from build123d import *

# Parameters (mm, degrees)
SKETCH_2_W          = 10
SKETCH_2_H          = 8
EXTRUDE_1_DEPTH     = 12.5
SKETCH_3_W          = 10
SKETCH_3_H          = 5
CUT_EXTRUDE_1_DEPTH = 10
SKETCH_4_R          = 1.6
CUT_EXTRUDE_2_DEPTH = 18.895530168
SKETCH_5_OUTSIDE_W  = 15.58
SKETCH_5_OUTSIDE_H  = 18.08
CUT_EXTRUDE_3_DEPTH = 18.895530168


with BuildPart() as part:
    # ｽｹｯﾁ2 → ﾎﾞｽ - 押し出し1 (new body)
    with BuildSketch(Plane(origin=(0, 0, 0), x_dir=(1, 0, 0), z_dir=(0, 1, 0))):
        with Locations((5, 4)):
            Rectangle(SKETCH_2_W, SKETCH_2_H)
    extrude(amount=EXTRUDE_1_DEPTH)

    # ｽｹｯﾁ3 → ｶｯﾄ - 押し出し1 (cut)
    with BuildSketch(Plane(origin=(0, 12.5, 0), x_dir=(1, 0, 0), z_dir=(0, 1, 0))):
        with Locations((5, 4)):
            Rectangle(SKETCH_3_W, SKETCH_3_H)
    extrude(amount=-CUT_EXTRUDE_1_DEPTH, mode=Mode.SUBTRACT)

    # ｽｹｯﾁ4 → ｶｯﾄ - 押し出し2 (cut, through all)
    with BuildSketch(Plane.XY):
        with Locations((5, 7.5)):
            Circle(SKETCH_4_R)
    extrude(amount=-CUT_EXTRUDE_2_DEPTH, mode=Mode.SUBTRACT)

    # ｽｹｯﾁ5 outside → ｶｯﾄ - 押し出し3 (cut, through all)
    with BuildSketch(Plane.XY):
        with Locations((5, 6.25)):
            Rectangle(SKETCH_5_OUTSIDE_W, SKETCH_5_OUTSIDE_H)
        with BuildLine():
            Line((0, 7.5), (0, 0))
            Line((0, 0), (10, 0))
            Line((10, 0), (10, 7.5))
            ThreePointArc((10, 7.5), (5, 12.5), (0, 7.5))
        make_face(mode=Mode.SUBTRACT)
    extrude(amount=-CUT_EXTRUDE_3_DEPTH, mode=Mode.SUBTRACT)


solid = part.part
Geometry: final body of the model. Coordinates: model frame, mm. A direction names the side the tool comes from. Give positions to 0.01 mm unless a question says otherwise; leave off trailing zeros. Write each loop counter-clockwise with the first axis right and the second up, starting at its lowest first coordinate (ties: lowest second). Pieces come first, ordered by that corner, then holes. Notation, with made-up numbers: (-1.5, -24) -> (53.5, -24) arc R26 cw to (53.5, 0) -> close; hole circle Ø7 at (4, 0). An arc over 180 degrees is marked (long way). Answer in a Markdown table with one row per item.
(1) Ray query, line 1 along Z through (x, y) = (1.25, 10.25); line 2 along Y through (x, z) = (5, -0.35); line 3 along Y through (x, z) = (1.75, -4). Return the intervals inside material, ascending. Write a range as [from, to].
Answers below:
| item | result |
|---|---|
| line 1 | [-8, -6.5], [-1.5, 0] |
| line 2 | [0, 5.9], [9.1, 12.5] |
| line 3 | [0, 2.5] |
(2) Draft query along X for faces 1 (the cylindrical face through (4.65, 5.94, -7.24)), 2 (the cylindrical face through (4.65, 5.94, -0.74)), 3 (the cylindrical face through (5.1, 12.5, -0.7)), 4 (the flat face through (5, 5, -6.5)). Return one class per face: +X half, -X half, draft (parallel to the pull), parting line (faces both ways), or undercut.
Answers below:
| item | result |
|---|---|
| face 1 | undercut |
| face 2 | undercut |
| face 3 | parting line |
| face 4 | draft |
(3) Set-up query: faces 5 (the flat face through (5, 5, -1.5)), 6 (the flat face through (5, 5, -8)). Return all of +Z, -Z, +X, -X, +Y, -Y with unobstructed straight access to the full face (end or side cutting, diameter ignored); none if empty.
Answers below:
| item | result |
|---|---|
| face 5 | +X, -X, +Y |
| face 6 | -Z, +X, -X, +Y, -Y |
(4) Section query D-D on x = 8. Return loops of the section in (y, z).
Answers below:
| item | result |
|---|---|
| outline | (0, -8) -> (11.5, -8) -> (11.5, -6.5) -> (2.5, -6.5) -> (2.5, -1.5) -> (11.5, -1.5) -> (11.5, 0) -> (0, 0) -> close |
(5) Section query B-B on x = 5. Return loops of the section in (y, z), then the cut area to 3 significant figures.
Answers below:
| item | result |
|---|---|
| outline | (0, -8) -> (5.9, -8) -> (5.9, -6.5) -> (2.5, -6.5) -> (2.5, -1.5) -> (5.9, -1.5) -> (5.9, 0) -> (0, 0) -> close; (9.1, -8) -> (12.5, -8) -> (12.5, -6.5) -> (9.1, -6.5) -> close; (9.1, -1.5) -> (12.5, -1.5) -> (12.5, 0) -> (9.1, 0) -> close |
| area | 40.4 mm^2 |
(6) Section query A-A on y = 3.25. Return loops of the section in (x, z).
Answers below:
| item | result |
|---|---|
| outline | (0, -8) -> (10, -8) -> (10, -6.5) -> (0, -6.5) -> close; (0, -1.5) -> (10, -1.5) -> (10, 0) -> (0, 0) -> close |
(7) Pin query (flat end, axial travel): pin 1 (3 mm diameter, centred on x = 5, y = 7.5, fed in from -Z); pin 2 (3 mm diameter, centred on y = 10, z = -2, fed in from +X). Return the tip coordinate at first contact, or that it passes through.
Answers below:
| item | result |
|---|---|
| pin 1 | through |
| pin 2 | x = 9.88 |
(8) Section query C-C on y = 6.5. Return loops of the section in (x, z).
Answers below:
| item | result |
|---|---|
| outline | (0, -8) -> (3.75, -8) -> (3.75, -6.5) -> (0, -6.5) -> close; (0, -1.5) -> (3.75, -1.5) -> (3.75, 0) -> (0, 0) -> close; (6.25, -8) -> (10, -8) -> (10, -6.5) -> (6.25, -6.5) -> close; (6.25, -1.5) -> (10, -1.5) -> (10, 0) -> (6.25, 0) -> close |
